The model under review builds one solid part; all positions refer to its coordinate system, in mm. A direction names the side the tool comes from. Round coordinates to 2 decimals unless told otherwise and drop trailing zeros. Write each loop counter-clockwise with the first axis right and the second up, starting at its lowest first coordinate (ties: lowest second). Pieces come first, ordered by that corner, then holes. Notation, with made-up numbers: M -35.75,61 L -28.75,61 A24 cw -28.75,89 Z; hole C -14,24 d10. An arc over 180 degrees is marked long. One line per item, written item: value. Start each with the question number.
1) Tool access review of faces 1 (the face through (-3.448, 16.802, 5.948)), 2 (the face through (5.48, 16.8, 3.21)), 3 (the face through (-6.875, 16.802, -0.013)), 4 (the face through (0, 11, 4.89)): name each direction out of +Z, -Z, +X, -X, +Y, -Y from which nothing blocks a thin tool from reaching the whole face with its end or side.
2) For P1, Ø8, axis at x = -1.5, y = 19, coming from the -Z side; P2, Ø1.7, axis at x = -1, y = 15.5, coming from the +Z side; P3, Ø2, axis at y = 3, z = 4.5, coming from the -X side, all flat-tipped, find the tip position at first contact; note any pin that passes through.
3) Take a section at B-B, the plane z = -2.25. Write out the cut boundary in (x, y).
4) Wall thickness on probe 1 along Z at (x, y) = (-0.75, 22); probe 2 along Y at (x, z) = (2, -6.5); probe 3 along Z at (x, y) = (-3.25, 9.5): over which ranges is each line inside the solid? List them lowest first.
from build123d import *

# Parameters (mm, degrees)
SKETCH1_R           = 9.525
BOSS_EXTRUDE1_DEPTH = 10.541
BOSS_EXTRUDE2_DEPTH = 12.7


with BuildPart() as part:
    # Sketch1 → Boss-Extrude1 (new body)
    with BuildSketch(Plane(origin=(0, 0, 0), x_dir=(1, 0, 0), z_dir=(0, 1, 0))):
        with Locations(Location((0, 0, 0), (0, 0, 270))):
            Circle(SKETCH1_R)
        Polygon((5.645908282, 0), (2.822954141, 4.8895), (-2.822954141, 4.8895), (-5.645908282, 0), (-2.822954141, -4.8895), (2.822954141, -4.8895), align=None, mode=Mode.SUBTRACT)
    extrude(amount=BOSS_EXTRUDE1_DEPTH)

    # Sketch2 → Boss-Extrude2 (add)
    with BuildSketch(Plane(origin=(0, 10.541, 0), x_dir=(1, 0, 0), z_dir=(0, 1, 0))):
        with BuildLine():
            Line((4.181770802, -5.456960506), (6.816751826, -0.893039494))
            ThreePointArc((6.816751826, -0.893039494), (6.875, 0), (6.816751826, 0.893039494))
            Line((6.816751826, 0.893039494), (4.181770802, 5.456960506))
            ThreePointArc((4.181770802, 5.456960506), (3.4375, 5.953924651), (2.634981025, 6.35))
            Line((2.634981025, 6.35), (-2.634981025, 6.35))
            ThreePointArc((-2.634981025, 6.35), (-3.4375, 5.953924651), (-4.181770802, 5.456960506))
            Line((-4.181770802, 5.456960506), (-6.816751826, 0.893039494))
            ThreePointArc((-6.816751826, 0.893039494), (-6.875, 0), (-6.816751826, -0.893039494))
            Line((-6.816751826, -0.893039494), (-4.181770802, -5.456960506))
            ThreePointArc((-4.181770802, -5.456960506), (-3.4375, -5.953924651), (-2.634981025, -6.35))
            Line((-2.634981025, -6.35), (2.634981025, -6.35))
            ThreePointArc((2.634981025, -6.35), (3.4375, -5.953924651), (4.181770802, -5.456960506))
        make_face()
        Polygon((-2.822954141, 4.8895), (2.822954141, 4.8895), (5.645908282, 0), (2.822954141, -4.8895), (-2.822954141, -4.8895), (-5.645908282, 0), align=None, mode=Mode.SUBTRACT)
    extrude(amount=BOSS_EXTRUDE2_DEPTH)


solid = part.part
Checked values:
1. face 1: +Z, -X, +Y
1. face 2: +Z, +X, +Y
1. face 3: -X, +Y
1. face 4: +Y, -Y
2. P1: stops at z = -6.35
2. P2: stops at z = 6.35
2. P3: stops at x = -8.86
3. outline: M -9.26,0 L -4.35,0 L -4.35,23.24 L -6.03,23.24 L -6.03,10.54 L -9.26,10.54 Z; M 4.35,0 L 9.26,0 L 9.26,10.54 L 6.03,10.54 L 6.03,23.24 L 4.35,23.24 Z
4. probe 1: z = -6.35 to -4.89, 4.89 to 6.35
4. probe 2: y = 0 to 10.54
4. probe 3: z = -8.95 to -4.15, 4.15 to 8.95
